Model file for the job. Use its own axes, mm. Give positions to 0.01 mm unless a question says otherwise; leave off trailing zeros. Write each loop counter-clockwise with the first axis right and the second up, starting at its lowest first coordinate (ties: lowest second). Pieces come first, ordered by that corner, then holes.
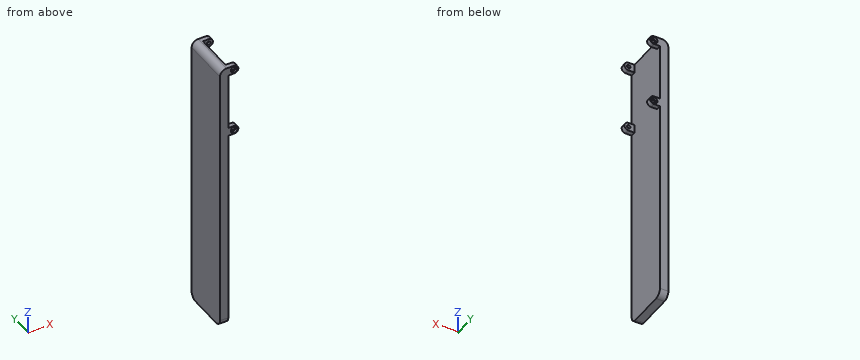
```python
from build123d import *

# Parameters (mm, degrees)
SKETCH1_W           = 5
SKETCH1_H           = 166
BOSS_EXTRUDE1_DEPTH = 29
SKETCH2_W           = 5
SKETCH2_H           = 2.9
BOSS_EXTRUDE2_DEPTH = 6
SKETCH3_R           = 1.05
CUT_EXTRUDE1_DEPTH  = 169.620876525
SKETCH4_R           = 2
CUT_EXTRUDE2_DEPTH  = 1.4
FILLET1_R           = 4
FILLET2_R           = 2.5


with BuildPart() as part:
    # Sketch1 → Boss-Extrude1 (new body)
    with BuildSketch(Plane(origin=(0, 0, 0), x_dir=(1, 0, 0), z_dir=(0, 1, 0))):
        with Locations((-2.5, 83)):
            Rectangle(SKETCH1_W, SKETCH1_H)
    extrude(amount=BOSS_EXTRUDE1_DEPTH)

    # Sketch2 → Boss-Extrude2 (add)
    with BuildSketch(Plane(origin=(0, 0, 0), x_dir=(0, 0, -1), z_dir=(1, 0, 0))):
        with Locations((2.5, 27.55)):
            Rectangle(SKETCH2_W, SKETCH2_H)
        with Locations((41.5, 27.55)):
            Rectangle(SKETCH2_W, SKETCH2_H)
        with Locations((41.5, 1.45)):
            Rectangle(SKETCH2_W, SKETCH2_H)
        with Locations((2.5, 1.45)):
            Rectangle(SKETCH2_W, SKETCH2_H)
    extrude(amount=BOSS_EXTRUDE2_DEPTH)

    # Sketch3 → Cut-Extrude1 (cut, through all)
    with BuildSketch(Plane(origin=(0, 29, 0), x_dir=(1, 0, 0), z_dir=(0, 1, 0))):
        with Locations(Location((3.5, 41.5, 0), (0, 0, 270))):
            Circle(SKETCH3_R)
        with Locations(Location((3.5, 2.5, 0), (0, 0, 270))):
            Circle(SKETCH3_R)
    extrude(amount=-CUT_EXTRUDE1_DEPTH, mode=Mode.SUBTRACT)

    # Sketch4 → Cut-Extrude2 (cut)
    with BuildSketch(Plane(origin=(0, 29, 0), x_dir=(1, 0, 0), z_dir=(0, 1, 0))):
        with Locations(Location((3.5, 41.5, 0), (0, 0, 270))):
            Circle(SKETCH4_R)
        with Locations(Location((3.5, 2.5, 0), (0, 0, 270))):
            Circle(SKETCH4_R)
    cut_extrude2 = extrude(amount=-CUT_EXTRUDE2_DEPTH, mode=Mode.SUBTRACT)

    # Mirror2: Cut-Extrude2 across plane
    add(cut_extrude2.mirror(Plane.ZX.offset(14.5)), mode=Mode.SUBTRACT)

    # Fillet1
    fillet1_edges = [part.edges().sort_by_distance(p)[0] for p in [
        (-2.5, 0, -166),
        (-5, 14.5, 0),
        (-2.5, 29, -166),
    ]]
    fillet(fillet1_edges, radius=FILLET1_R)

    # Fillet2
    fillet2_edges = [part.edges().sort_by_distance(p)[0] for p in [
        (6, 1.45, -5),
        (6, 1.45, 0),
        (6, 1.45, -44),
        (6, 1.45, -39),
        (6, 27.55, -44),
        (6, 27.55, -39),
        (6, 27.55, -5),
        (6, 27.55, 0),
    ]]
    fillet(fillet2_edges, radius=FILLET2_R - 0.0001)  # a hair under: the kernel refuses the full size


solid = part.part
```
1. Pin check, flat tips, straight feed: P1, Ø2.5, axis at x = 3.5, z = -41.5, coming from the -Y side; P2, Ø3, axis at x = 3.5, z = -41.5, coming from the +Y side; P3, Ø1.4, axis at x = 1.5, y = 1, coming from the -Z side. Stop position of each tip, or through.
Calculated:
P1: stops at y = 1.4
P2: stops at y = 27.6
P3: stops at z = -44
2. Slice it at B-B, the plane z = -149. Write the cut outline in (x, y).
Calculated:
outline: (-5, 0) - (0, 0) - (0, 29) - (-5, 29) - close
3. Slice it at A-A, the plane y = 15.75. Write the cut outline in (x, z).
Calculated:
outline: (-5, -166) - (0, -166) - (0, 0) - (-1, 0) arc R4 ccw to (-5, -4) - close
4. Probe probe 1 along X at (y, z) = (2.55, -41.5); probe 2 along X at (y, z) = (0.95, -41.5); probe 3 along X at (y, z) = (9.5, -158.5). List the from-to ranges inside material, lowest first.
Calculated:
probe 1: x = -5 to 2.45, 4.55 to 6
probe 2: x = -5 to 1.5, 5.5 to 6
probe 3: x = -5 to 0
